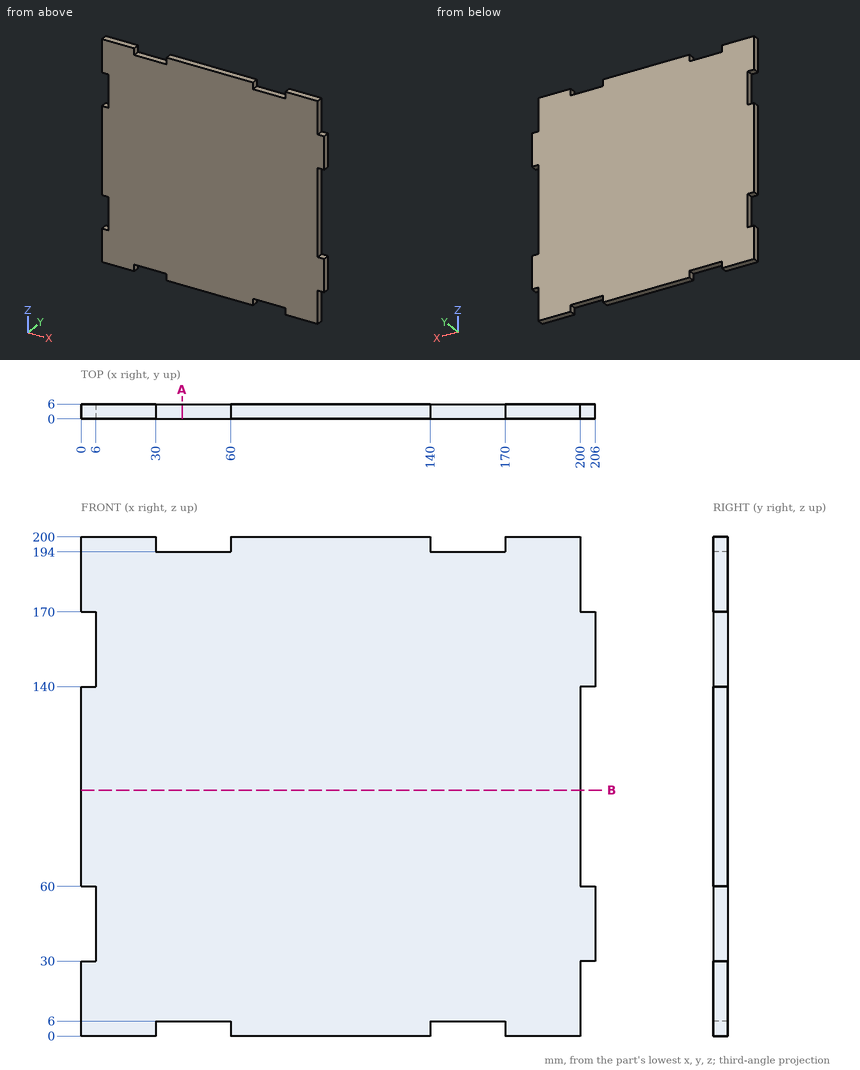
Could you check a few things on this drawing? It's one solid part, dimensions in mm from its lowest x, y, z. Give positions to 0.01 mm unless a question says otherwise; leave off trailing zeros. Order: outer loops, then holes, each group sorted by start corner. A loop starts at its lowest first (then second) coordinate and runs counter-clockwise, first axis right, second up. Notation, with made-up numbers: (11, 6.5) - (30, 6.5) arc R18 cw to (30, 10.5) - close; hole circle Ø1 at (34, 0). An arc over 180 degrees is marked (long way). Answer as a JSON object with one key per item and string values. Group by question number.
Item 1: For P1, Ø1, axis at y = 1.5, z = 73.5, coming from the +X side; P2, Ø3, axis at y = 2.5, z = 153, coming from the -X side; P3, Ø3, axis at x = 156.5, y = 2.5, coming from the +Z side, each with a flat end and sliding along its axis, tell me the tip position at first contact or that it passes through.
Item 2: If we section it at B-B on z = 98.5: Please give me the cut outline in (x, y), and give its area (3 significant figures).
Item 3: If we section it at A-A on x = 40.5: Please give me the cut outline in (y, z), and give its area (3 significant figures).
Item 4: Please list where these lines run through material, in increasing order: probe 1 along X at (y, z) = (2.95, 105); probe 2 along Z at (x, y) = (154, 2.1); probe 3 along X at (y, z) = (0.75, 142).
Result set:
{
 "1": {"P1": "x = 200", "P2": "x = 6", "P3": "z = 194"},
 "2": {"outline": "(0, 0) - (200, 0) - (200, 6) - (0, 6) - close", "area": "1,200 mm²"},
 "3": {"outline": "(0, 6) - (6, 6) - (6, 194) - (0, 194) - close", "area": "1,130 mm²"},
 "4": {"probe 1": "0 to 200", "probe 2": "6 to 194", "probe 3": "6 to 206"}
}
